from build123d import *

# Parameters (mm, degrees)
F0_W           = 90
F0_H           = 90
F0_W_2         = 70.5104
F0_H_2         = 29.0068
F0_W_3         = 70.5
F0_H_3         = 29
F1_DEPTH       = 4
F3_D           = 3
F3_CSINK_D     = 6
F3_CSINK_ANGLE = 90
F4_T1_DEPTH    = 88
F4_T3_DEPTH    = 88
F4_T5_DEPTH    = 5.5
F4_S9_W        = 1
F4_S9_H        = 1
F4_T10_DEPTH   = 1
F4_S15_W       = 1
F4_S15_H       = 1
F4_T16_DEPTH   = 1
F4_S21_W       = 1
F4_S21_H       = 1
F4_T22_DEPTH   = 1
F4_S27_W       = 1
F4_S27_H       = 1
F4_T28_DEPTH   = 1


# Not quite as in the source:
# - a fillet or chamfer that OpenCascade refuses, or shapes differently, is made with other operations: its cross-section is extruded or revolved along the edge and cut away or added


with BuildPart() as f1:
    # F0 (on Top) → F1 (new body)
    with BuildSketch(Plane.XY):
        Rectangle(F0_W, F0_H)
        with Locations((-0.2552, -20.4966)):
            Rectangle(F0_W_2, F0_H_2, mode=Mode.SUBTRACT)
        with Locations((-0.25, 20.5)):
            Rectangle(F0_W_3, F0_H_3, mode=Mode.SUBTRACT)
    extrude(amount=F1_DEPTH)

    # F3 (through all)
    with Locations(Plane.XY.offset(4)):
        with Locations((-41, 41), (41, 41), (41, -41), (-41, -41)):
            CounterSinkHole(F3_D / 2, F3_CSINK_D / 2, counter_sink_angle=F3_CSINK_ANGLE)

    # F4: fillet of radius 1 on 8 edges, made by hand

    # F4_s2 → F4_t1 (cut)
    with BuildSketch(Plane.YZ.offset(-44)):
        with BuildLine():
            ThreePointArc((45, 3), (44.7071067812, 3.7071067812), (44, 4))
            Line((44, 4), (45, 4))
            Line((45, 4), (45, 3))
        make_face()
        with BuildLine():
            ThreePointArc((-44, 4), (-44.7071067812, 3.7071067812), (-45, 3))
            Line((-45, 3), (-45, 4))
            Line((-45, 4), (-44, 4))
        make_face()
    extrude(amount=F4_T1_DEPTH, mode=Mode.SUBTRACT)

    # F4_s4 → F4_t3 (cut)
    with BuildSketch(Plane.XZ.offset(-44)):
        with BuildLine():
            ThreePointArc((-45, 3), (-44.7071067812, 3.7071067812), (-44, 4))
            Line((-44, 4), (-45, 4))
            Line((-45, 4), (-45, 3))
        make_face()
        with BuildLine():
            ThreePointArc((45, 3), (44.7071067812, 3.7071067812), (44, 4))
            Line((44, 4), (45, 4))
            Line((45, 4), (45, 3))
        make_face()
    extrude(amount=F4_T3_DEPTH, mode=Mode.SUBTRACT)

    # F4_s6 → F4_t5 (cut)
    with BuildSketch(Plane.XY.offset(-2.5)):
        with BuildLine():
            ThreePointArc((45, -44), (44.7071067812, -44.7071067812), (44, -45))
            Line((44, -45), (45, -45))
            Line((45, -45), (45, -44))
        make_face()
        with BuildLine():
            ThreePointArc((44, 45), (44.7071067812, 44.7071067812), (45, 44))
            Line((45, 44), (45, 45))
            Line((45, 45), (44, 45))
        make_face()
        with BuildLine():
            ThreePointArc((-44, 45), (-44.7071067812, 44.7071067812), (-45, 44))
            Line((-45, 44), (-45, 45))
            Line((-45, 45), (-44, 45))
        make_face()
        with BuildLine():
            ThreePointArc((-45, -44), (-44.7071067812, -44.7071067812), (-44, -45))
            Line((-44, -45), (-45, -45))
            Line((-45, -45), (-45, -44))
        make_face()
    extrude(amount=F4_T5_DEPTH, mode=Mode.SUBTRACT)


with BuildPart() as f4_tool8:
    # F4_s9 → F4_t10 (new body)
    with BuildSketch(Plane.XZ.offset(-44)):
        with Locations((44.5, 3.5)):
            Rectangle(F4_S9_W, F4_S9_H)
    extrude(amount=-F4_T10_DEPTH)

    # F4_s11 → F4_t12 (revolve, cut)
    with BuildSketch(Plane(origin=(44, 44, 3), x_dir=(-0.7071067812, 0, -0.7071067812), z_dir=(0.7071067812, 0, -0.7071067812))):
        with BuildLine():
            ThreePointArc((0, -1), (1, 0), (0, 1))
            Line((0, 1), (0, -1))
        make_face()
    revolve(axis=Axis((44, 44, 3), (0, 1, 0)), mode=Mode.SUBTRACT)


with BuildPart() as f1_1:
    add(f1.part)

    # F4_t7: cut F4_tool8
    add(f4_tool8.part, mode=Mode.SUBTRACT)


with BuildPart() as f4_tool14:
    # F4_s15 → F4_t16 (new body)
    with BuildSketch(Plane.XZ.offset(-44)):
        with Locations((-44.5, 3.5)):
            Rectangle(F4_S15_W, F4_S15_H)
    extrude(amount=-F4_T16_DEPTH)

    # F4_s17 → F4_t18 (revolve, cut)
    with BuildSketch(Plane(origin=(-44, 44, 3), x_dir=(0.7071067812, 0, -0.7071067812), z_dir=(0.7071067812, 0, 0.7071067812))):
        with BuildLine():
            ThreePointArc((0, -1), (1, 0), (0, 1))
            Line((0, 1), (0, -1))
        make_face()
    revolve(axis=Axis((-44, 44, 3), (0, 1, 0)), mode=Mode.SUBTRACT)


with BuildPart() as f1_2:
    add(f1_1.part)

    # F4_t13: cut F4_tool14
    add(f4_tool14.part, mode=Mode.SUBTRACT)


with BuildPart() as f4_tool20:
    # F4_s21 → F4_t22 (new body)
    with BuildSketch(Plane.YZ.offset(-44)):
        with Locations((-44.5, 3.5)):
            Rectangle(F4_S21_W, F4_S21_H)
    extrude(amount=-F4_T22_DEPTH)

    # F4_s23 → F4_t24 (revolve, cut)
    with BuildSketch(Plane(origin=(-44, -44, 3), x_dir=(0, 0.7071067812, -0.7071067812), z_dir=(0, 0.7071067812, 0.7071067812))):
        with BuildLine():
            ThreePointArc((0, -1), (1, 0), (0, 1))
            Line((0, 1), (0, -1))
        make_face()
    revolve(axis=Axis((-44, -44, 3), (-1, 0, 0)), mode=Mode.SUBTRACT)


with BuildPart() as f1_3:
    add(f1_2.part)

    # F4_t19: cut F4_tool20
    add(f4_tool20.part, mode=Mode.SUBTRACT)


with BuildPart() as f4_tool26:
    # F4_s27 → F4_t28 (new body)
    with BuildSketch(Plane.YZ.offset(44)):
        with Locations((-44.5, 3.5)):
            Rectangle(F4_S27_W, F4_S27_H)
    extrude(amount=F4_T28_DEPTH)

    # F4_s29 → F4_t30 (revolve, cut)
    with BuildSketch(Plane(origin=(44, -44, 3), x_dir=(0, 0.7071067812, -0.7071067812), z_dir=(0, -0.7071067812, -0.7071067812))):
        with BuildLine():
            ThreePointArc((0, -1), (1, 0), (0, 1))
            Line((0, 1), (0, -1))
        make_face()
    revolve(axis=Axis((44, -44, 3), (1, 0, 0)), mode=Mode.SUBTRACT)


with BuildPart() as f1_4:
    add(f1_3.part)

    # F4_t25: cut F4_tool26
    add(f4_tool26.part, mode=Mode.SUBTRACT)


solid = f1_4.part
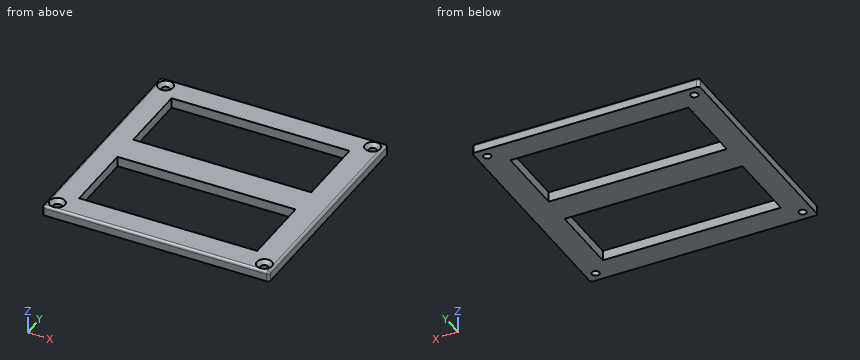
Design review of the part built by this model. Coordinates are the model's own, in mm. Coordinates: 2 decimals unless noted, no trailing zeros. Loops run counter-clockwise (first coordinate to the right, second up) from the corner with the lowest first, then second, coordinate; pieces in that order, holes last. Notation, with made-up numbers: (-19.75, -23) -> (19.25, -23) arc R22 cw to (19.25, -7) -> close; hole circle Ø4 at (84.25, -4.75). An arc over 180 degrees is marked (long way). Use a Markdown table: item, result. Add a question column.
Item 1: Wall thickness on L1, parallel to Y at x = -9.5, z = 2.4; L2, parallel to Y at x = -41, z = 1.9: over which ranges is each line inside the solid? List them lowest first. Write a range as from..to.
Item 2: We need section B-B, the plane x = -32. Write out the cut boundary in (y, z), and give its area (3 significant figures).
Item 3: We need section D-D, the plane y = -12.5. Write out the cut boundary in (x, z).
Item 4: We need section C-C, the plane z = 1.8. Write out the cut boundary in (x, y).
Item 5: We need section A-A, the plane y = 13. Write out the cut boundary in (x, z), and give its area (3 significant figures).
Numbers:
| question | item | result |
|---|---|---|
| 1 | L1 | y = -45..-35, -5.99..6, 35..45 |
| 1 | L2 | y = -45..-42.5, -39.5..39.5, 42.5..45 |
| 2 | outline | (-45, 0) -> (-35, 0) -> (-35, 4) -> (-44, 4) arc R1 ccw to (-45, 3) -> close; (-5.99, 0) -> (6, 0) -> (6, 4) -> (-5.99, 4) -> close; (35, 0) -> (45, 0) -> (45, 3) arc R1 ccw to (44, 4) -> (35, 4) -> close |
| 2 | area | 128 mm^2 |
| 3 | outline | (-45, 0) -> (-35.51, 0) -> (-35.51, 4) -> (-44, 4) arc R1 ccw to (-45, 3) -> close; (35, 0) -> (45, 0) -> (45, 3) arc R1 ccw to (44, 4) -> (35, 4) -> close |
| 4 | outline | (-45, -44) arc R1 ccw to (-44, -45) -> (44, -45) arc R1 ccw to (45, -44) -> (45, 44) arc R1 ccw to (44, 45) -> (-44, 45) arc R1 ccw to (-45, 44) -> close; hole circle Ø3 at (-41, -41); hole circle Ø3 at (-41, 41); hole (-35.51, -35) -> (35, -35) -> (35, -5.99) -> (-35.51, -5.99) -> close; hole (-35.5, 6) -> (35, 6) -> (35, 35) -> (-35.5, 35) -> close; hole circle Ø3 at (41, -41); hole circle Ø3 at (41, 41) |
| 5 | outline | (-45, 0) -> (-35.5, 0) -> (-35.5, 4) -> (-44, 4) arc R1 ccw to (-45, 3) -> close; (35, 0) -> (45, 0) -> (45, 3) arc R1 ccw to (44, 4) -> (35, 4) -> close |
| 5 | area | 77.6 mm^2 |
